from build123d import *

# Parameters (mm, degrees)
HEXAGONSOCKET_DEPTH = 1.5
HEADFILLET_R        = 0.2
CHAMFER_2_SIZE      = 0.379
SKETCH4_W           = 5
SKETCH4_H           = 5


with BuildPart() as part:
    # Sketch1 → Base (revolve)
    with BuildSketch(Plane.XY, mode=Mode.PRIVATE) as base_sk:
        Polygon((0, 0), (0, 4.48), (2.48, 2), (10, 2), (10, 0), align=None)
    revolve(base_sk.sketch.rotate(Axis((-0.587069181, 0, 0), (1, 0, 0)), 90), axis=Axis((-0.587069181, 0, 0), (1, 0, 0)))

    # Sketch2 → HexagonSocket (cut)
    with BuildSketch(Plane(origin=(0, 0, 0), x_dir=(0, 0, -1), z_dir=(1, 0, 0))):
        Polygon((1.443375673, 0), (0.721687836, 1.25), (-0.721687836, 1.25), (-1.443375673, 0), (-0.721687836, -1.25), (0.721687836, -1.25), align=None)
    extrude(amount=HEXAGONSOCKET_DEPTH, mode=Mode.SUBTRACT)

    # Sketch3 → Cut-Revolve1 (revolve, cut)
    with BuildSketch(Plane.XY, mode=Mode.PRIVATE) as cut_revolve1_sk:
        Polygon((1.5, 1.25), (2.221687836, 0), (1.5, 0), align=None)
    revolve(cut_revolve1_sk.sketch.rotate(Axis((-0.439109555, 0, 0), (1, 0, 0)), 90), axis=Axis((-0.439109555, 0, 0), (1, 0, 0)), mode=Mode.SUBTRACT)

    # HeadFillet
    headfillet_edges = [part.edges().sort_by_distance(p)[0] for p in [
        (2.48, 0, -2),
    ]]
    fillet(headfillet_edges, radius=HEADFILLET_R)

    # Chamfer 2
    chamfer_2_edges = [part.edges().sort_by_distance(p)[0] for p in [
        (10, 0, -2),
    ]]
    chamfer(chamfer_2_edges, length=CHAMFER_2_SIZE)

    # Sketch4 → Cut-Revolve2 (revolve, cut)
    with BuildSketch(Plane(origin=(0, 0, 0), x_dir=(1, 0, 0), z_dir=(0, 1, 0)), mode=Mode.PRIVATE) as cut_revolve2_sk:
        with Locations((0.5, 6.265)):
            Rectangle(SKETCH4_W, SKETCH4_H)
    revolve(cut_revolve2_sk.sketch.rotate(Axis((11.853138686, 0, 0), (-1, 0, 0)), 180), axis=Axis((11.853138686, 0, 0), (-1, 0, 0)), mode=Mode.SUBTRACT)


solid = part.part
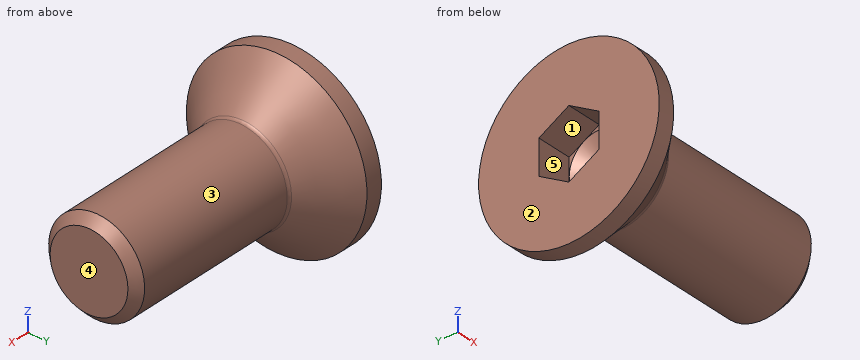
Geometry check sheet. Reference: the model listing, model coordinates, mm. Face numbers are marked on the shaded views. A direction names the side the tool comes from. Give positions to 0.01 mm unless a question says otherwise; leave off trailing zeros. Order: outer loops, then holes, each group sorted by start corner. A loop starts at its lowest first (then second) coordinate and runs counter-clockwise, first axis right, second up. Notation, with made-up numbers: (-19, 13) - (-7, 13) arc R33 ccw to (-7, 50) - close; hole circle Ø10 at (1.25, 53.25). An arc over 180 degrees is marked (long way). Answer as a JSON object with one key per item and string values.
(1) Material ranges on line 1 (X direction, y = -2.25, z = -1.5); line 2 (Y direction, x = 4.75, z = -1.5); line 3 (Z direction, x = 6.25, y = -1.25), recorded low to high.
Report:
{"line 1": "0 to 1.78", "line 2": "-1.32 to 1.32", "line 3": "-1.56 to 1.56"}
(2) Tool access check on the marked faces 1 and 2. Record the directions out of +Z, -Z, +X, -X, +Y, -Y that give a thin tool (end or side, any length) a straight path to the whole face; none if there is none.
Report:
{"face 1": "-X", "face 2": "+Z, -Z, -X, +Y, -Y"}
(3) Depth check by flat-ended pin: pin 1 Ø4 at (x, y) = (3.5, 0.5) entering from -Z; pin 2 Ø0.7 at (x, z) = (1, -0.5) entering from +Y; pin 3 Ø1 at (x, y) = (8.5, 0.5) entering from -Z. Enter the tip coordinate at first touch or a pass-through.
Report:
{"pin 1": "z = -2.95", "pin 2": "y = 3.75", "pin 3": "z = -2"}
(4) Cross-section at B-B (x = 4.25). Record the cut outline in (y, z), then the cut area to 3 significant figures.
Report:
{"outline": "circle Ø4 at (0, 0)", "area": "12.6 mm^2"}
(5) Draft check along Y on the marked faces 3, 4 and 5. Enter one of: released by +Y, released by -Y, zero draft, split by the parting line, or undercut.
Report:
{"face 3": "split by the parting line", "face 4": "zero draft", "face 5": "undercut"}
(6) Cross-section at A-A (x = 1.25). Record the cut outline in (y, z).
Report:
{"outline": "circle Ø6.46 at (0, 0); hole (-1.25, -0.72) - (0, -1.44) - (1.25, -0.72) - (1.25, 0.72) - (0, 1.44) - (-1.25, 0.72) - close"}
